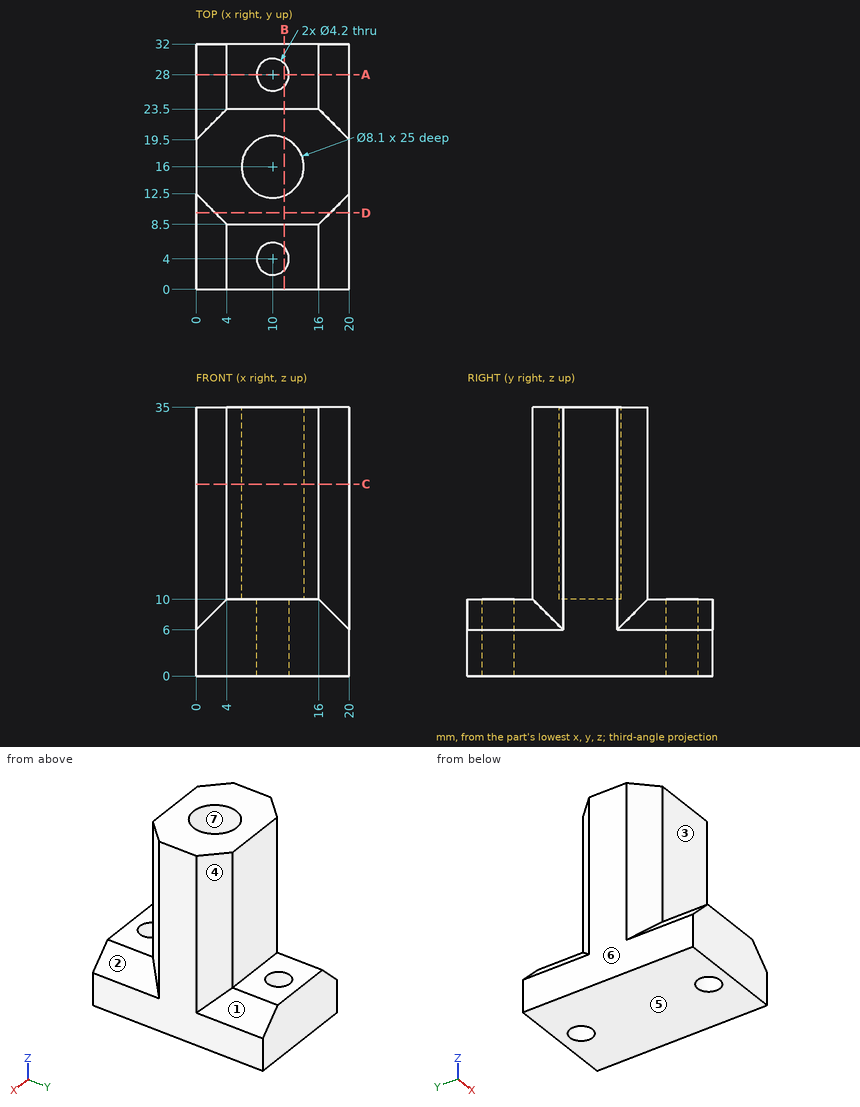
Part print with two shaded views. Sizes in mm from the minimum x, y, z corner. A direction names the side the tool comes from. Coordinates: 2 decimals unless noted, no trailing zeros. Loops run counter-clockwise (first coordinate to the right, second up) from the corner with the lowest first, then second, coordinate; pieces in that order, holes last. Notation, with made-up numbers: (-27, -29) -> (27, -29) arc R17 cw to (27, 3) -> close; hole circle Ø1 at (13, 5). An arc over 180 degrees is marked (long way). Answer as a JSON object with one key per item and string values.
Q1. Cut at A-A (y = 28). List the corners of the cut face in (x, z).
Report:
{"outline": "(0, 0) -> (7.9, 0) -> (7.9, 10) -> (4, 10) -> (0, 6) -> close; (12.1, 0) -> (20, 0) -> (20, 6) -> (16, 10) -> (12.1, 10) -> close"}
Q2. 3-axis set-ups, long thin cutter, end or side, ignore diameter. For the marked faces 1, 2 and 3: which of +Z, -Z, +X, -X, +Y, -Y reach the whole face in a straight line?
Report:
{"face 1": "+Z, +X, +Y", "face 2": "+Z, +X, -Y", "face 3": "+Z, +X, -X, -Y"}
Q3. Flat gauge pins, fed straight in: P1, Ø8, axis at x = 12.5, z = 31, coming from the -Y side; P2, Ø7, axis at x = 8.5, y = 3.5, coming from the +Z side; P3, Ø3, axis at x = 5.5, z = 22.5, coming from the +Y side; P4, Ø2.5, axis at x = 10, y = 28, coming from the +Z side. Where does each tip first touch, or does it go through?
Report:
{"P1": "stops at y = 8.5", "P2": "stops at z = 10", "P3": "stops at y = 23.5", "P4": "passes through"}
Q4. Cut at D-D (y = 10). List the corners of the cut face in (x, z), and give its area (3 significant figures).
Report:
{"outline": "(0, 0) -> (20, 0) -> (20, 6) -> (17.5, 8.5) -> (17.5, 35) -> (2.5, 35) -> (2.5, 8.5) -> (0, 6) -> close", "area": "561 mm2"}
Q5. Probe probe 1 along Y at (x, z) = (10, 2); probe 2 along Y at (x, z) = (10, 22.5); probe 3 along Z at (x, y) = (2.5, 30). List the from-to ranges inside material, lowest first.
Report:
{"probe 1": "y = 0 to 1.9, 6.1 to 25.9, 30.1 to 32", "probe 2": "y = 8.5 to 11.95, 20.05 to 23.5", "probe 3": "z = 0 to 8.5"}
Q6. Cut at C-C (z = 25). List the corners of the cut face in (x, y).
Report:
{"outline": "(0, 12.5) -> (4, 8.5) -> (16, 8.5) -> (20, 12.5) -> (20, 19.5) -> (16, 23.5) -> (4, 23.5) -> (0, 19.5) -> close; hole circle Ø8.1 at (10, 16)"}
Q7. Pull direction X, two halves, no side cores. Call the marked faces 4, 5, 6 and 7: released by +X, released by -X, zero draft, split by the parting line, or undercut.
Report:
{"face 4": "released by +X", "face 5": "zero draft", "face 6": "released by -X", "face 7": "undercut"}
Q8. Cut at B-B (x = 11.5). List the corners of the cut face in (y, z), and give its area (3 significant figures).
Report:
{"outline": "(0, 0) -> (2.53, 0) -> (2.53, 10) -> (0, 10) -> close; (5.47, 0) -> (26.53, 0) -> (26.53, 10) -> (23.5, 10) -> (23.5, 35) -> (19.76, 35) -> (19.76, 10) -> (12.24, 10) -> (12.24, 35) -> (8.5, 35) -> (8.5, 10) -> (5.47, 10) -> close; (29.47, 0) -> (32, 0) -> (32, 10) -> (29.47, 10) -> close", "area": "448 mm2"}
